Geometry: final body of the model. Coordinates: model frame, mm. Face numbers are marked on the shaded views. Coordinates: 2 decimals unless noted, no trailing zeros. Write each loop counter-clockwise with the first axis right and the second up, starting at its lowest first coordinate (ties: lowest second). Pieces come first, ordered by that corner, then holes. Notation, with made-up numbers: M 63,46.25 L 71,46.25 A12 cw 71,69.25 Z; hole C 36.5,-13 d1. An arc over 180 degrees is marked long. Write item = value, one per line. Start each with the question number.
Item 1: First-contact query: pin 1 Ø6 at (x, z) = (15, 3.5) entering from +Y; pin 2 Ø4 at (x, z) = (6, 6) entering from +Y; pin 3 Ø2 at (x, z) = (-6, 2.5) entering from -Y. Flat tips, straight axial feed; report the tip coordinate or a pass-through.
Item 2: Ray query, L1, parallel to Y at x = 0, z = 1.25; L2, parallel to Y at x = 4, z = 1.5; L3, parallel to X at y = 1.5, z = 3.5. Return the intervals inside material, ascending. Write a range as [from, to].
Item 3: Section D-D on x = -15.5. Output: boundary loops of the cut face in (y, z), plus the area to 3 significant figures.
Item 4: Section A-A on x = 0. Output: boundary loops of the cut face in (y, z).
Item 5: Section C-C on y = 4.5. Output: boundary loops of the cut face in (x, z), plus the area to 3 significant figures.
Item 6: Pull-direction query (X, two-part tool) for the marked faces 1, 2 and 3; classes: +X half, -X half, draft (parallel to the pull), parting line (faces both ways), or undercut.
Item 7: Section B-B on y = 0. Output: boundary loops of the cut face in (x, z).
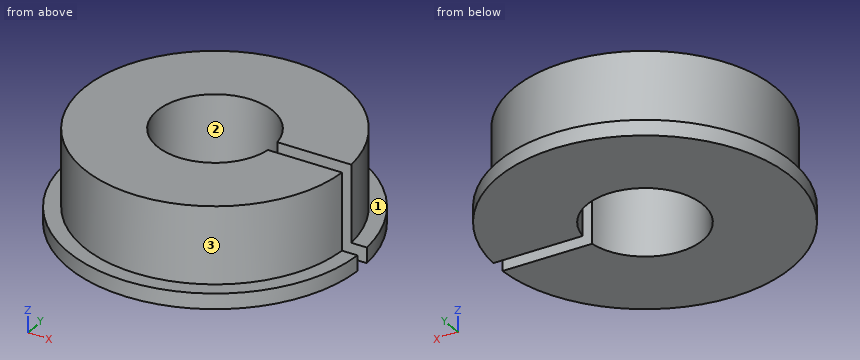
Autodesk Inventor part; units mm, degrees
ref_plane "YZ Plane" through (0, 0, 0) normal (1, 0, 0) x (0, 1, 0)
ref_plane "XZ Plane" through (0, 0, 0) normal (0, 1, 0) x (-1, 0, 0)
ref_plane "XY Plane" through (0, 0, 0) normal (0, 0, 1) x (1, 0, 0)
sketch "Skizze1" plane through (0, 0, 0) normal (0, 0, 1) x (1, 0, 0)
  arc A0 (7.433, 1) -> (7.433, -1) centre (0, 0) ccw
  arc A1 (16.9706, 1) -> (16.9706, -1) centre (0, 0) ccw
  line L0 (0, 0) -> (15.5172, 0) construction
  line L1 (7.433, -1) -> (16.9706, -1)
  line L2 (7.433, 1) -> (16.9706, 1)
  circle A2 centre (0, 0) radius 7.5 construction
  circle A3 centre (0, 0) radius 17 construction
  dimension "d0" = 15
  dimension "d1" = 34
  dimension "d2" = 2
extrude "Extrusion1" add sketch "Skizze1" along normal blind 10
sketch "Skizze2" plane through (0, 0, 0) normal (0, 0, -1) x (-1, 0, 0)
  arc A0 (-7.433, -1) -> (-7.433, 1) centre (0, 0) ccw
  line L0 (-7.433, -1) -> (-16.9706, -1)
  arc A1 (-16.9706, -1) -> (-16.9706, 1) centre (0, 0) ccw
  line L1 (-16.9706, 1) -> (-7.433, 1)
  arc A2 (-18.9737, -1) -> (-18.9737, 1) centre (0, 0) ccw
  line L2 (-16.9706, -1) -> (-18.9737, -1)
  line L3 (-16.9706, 1) -> (-18.9737, 1)
  dimension "d5" = 2
extrude "Extrusion2" add sketch "Skizze2" along normal blind 2
properties part number "edingClamp" material "ABS-Kunststoff"
Responses:
q1.pin_1 = 12.04
q1.pin_2 = 16.52
q1.pin_3 = -16.25
q2.L1 = [-17, -7.5], [7.5, 17]
q2.L2 = [-16.52, -6.34], [6.34, 16.52]
q2.L3 = [-16.93, -7.35], [7.35, 16.93]
q3.outline = M -10.99,-2 L 10.99,-2 L 10.99,0 L 6.98,0 L 6.98,10 L -6.98,10 L -6.98,0 L -10.99,0 Z
q3.area = 184 mm²
q4.outline = M -19,-2 L -7.5,-2 L -7.5,10 L -17,10 L -17,0 L -19,0 Z; M 7.5,-2 L 19,-2 L 19,0 L 17,0 L 17,10 L 7.5,10 Z
q5.outline = M -18.46,-2 L -6,-2 L -6,10 L -16.39,10 L -16.39,0 L -18.46,0 Z; M 6,-2 L 18.46,-2 L 18.46,0 L 16.39,0 L 16.39,10 L 6,10 Z
q5.area = 258 mm²
q6.face_1 = draft
q6.face_2 = undercut
q6.face_3 = parting line
q7.outline = M -19,-2 L -7.5,-2 L -7.5,10 L -17,10 L -17,0 L -19,0 Z
